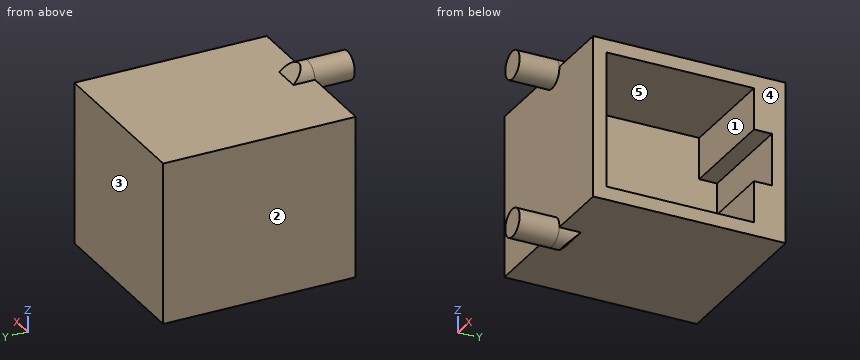
from build123d import *

# Parameters (mm, degrees)
SKETCH1_W           = 13
SKETCH1_H           = 12.2
BOSS_EXTRUDE1_DEPTH = 14.55
SKETCH2_R           = 1.05
BOSS_EXTRUDE2_DEPTH = 3
CUT_EXTRUDE1_DEPTH  = 8
CHAMFER1_SIZE       = 1.63


with BuildPart() as part:
    # Sketch1 → Boss-Extrude1 (new body)
    with BuildSketch(Plane(origin=(0, 0, 0), x_dir=(1, 0, 0), z_dir=(0, 1, 0))):
        with Locations((6.5, 6.1)):
            Rectangle(SKETCH1_W, SKETCH1_H)
    extrude(amount=BOSS_EXTRUDE1_DEPTH)

    # Sketch2 → Boss-Extrude2 (add)
    with BuildSketch(Plane.XZ):
        with Locations(Location((7, -0.1, 0), (0, 0, 174.5349762))):
            Circle(SKETCH2_R)
        with Locations(Location((7, -12.1, 0), (0, 0, 354.5349762))):
            Circle(SKETCH2_R)
    extrude(amount=BOSS_EXTRUDE2_DEPTH)

    # Sketch3 → Cut-Extrude1 (cut)
    with BuildSketch(Plane(origin=(13, 0, 0), x_dir=(0, 0, -1), z_dir=(1, 0, 0))):
        Polygon((1.000271868, 12.149637893), (1.000271868, 1.000271868), (11.199728132, 1.000271868), (11.199728132, 12.149637893), (8.065074736, 12.149637893), (8.065074736, 13.503489481), (4.134925264, 13.503489481), (4.134925264, 12.149637893), align=None)
    extrude(amount=-CUT_EXTRUDE1_DEPTH, mode=Mode.SUBTRACT)

    # Chamfer1
    # the kernel refuses this chamfer: 1.63 mm, written as the material it adds along each edge
    with BuildSketch(Plane(origin=(1.762929482, 0, 0), x_dir=(0, 0.9996219169112968, -0.027495876610586376), z_dir=(1, 0, 0))) as chamfer1_piece_1_section:
        Polygon((CHAMFER1_SIZE * 0.999621916911, CHAMFER1_SIZE * 0.0274958766106), (-CHAMFER1_SIZE * 0.0274958766106, CHAMFER1_SIZE * 0.999621916911), (0, 0), align=None)
    chamfer1_piece_1 = extrude(amount=10.474141037, mode=Mode.PRIVATE)
    chamfer1_piece_1 = chamfer1_piece_1 & Plane(origin=(7, 0.64054065, -0.1), x_dir=(-0.9954545219220755, 0, 0.09523809523973083), z_dir=(0, 1, 0)) * Cylinder(1.05, 28, mode=Mode.PRIVATE)
    add(chamfer1_piece_1)
    with BuildSketch(Plane(origin=(12.237070518, 0, -12.2), x_dir=(0, 0.9996219169112968, 0.02749587661058688), z_dir=(-1, 0, 0))) as chamfer1_piece_2_section:
        Polygon((CHAMFER1_SIZE * 0.999621916911, CHAMFER1_SIZE * 0.0274958766106), (-CHAMFER1_SIZE * 0.0274958766106, CHAMFER1_SIZE * 0.999621916911), (0, 0), align=None)
    chamfer1_piece_2 = extrude(amount=10.474141037, mode=Mode.PRIVATE)
    chamfer1_piece_2 = chamfer1_piece_2 & Plane(origin=(7, 0.64054065, -12.1), x_dir=(0.9954545219220756, 0, -0.09523809523973051), z_dir=(0, 1, 0)) * Cylinder(1.05, 28, mode=Mode.PRIVATE)
    add(chamfer1_piece_2)


solid = part.part
For this review, take the finished solid that the model builds, in its own axes (mm). Face numbers are marked on the shaded views. A direction names the side the tool comes from. Give positions to 0.01 mm unless a question says otherwise; leave off trailing zeros. Loops run counter-clockwise (first coordinate to the right, second up) from the corner with the lowest first, then second, coordinate; pieces in that order, holes last. Notation, with made-up numbers: (-22, 12) -> (0, 12) arc R11 ccw to (0, 30) -> close; hole circle Ø2 at (78.25, -21.75). An arc over 180 degrees is marked (long way). One line per question, with ' | ' between items.
1) We need section C-C (z = -8.75). Write out the cut boundary in (x, y), plus the area to 4 significant figures.
Resolved:
outline: (0, 0) -> (13, 0) -> (13, 1) -> (5, 1) -> (5, 12.15) -> (13, 12.15) -> (13, 14.55) -> (0, 14.55) -> close | area: 100.0 mm2
2) We need section A-A (x = 7). Write out the cut boundary in (y, z).
Resolved:
outline: (-3, -13.15) -> (0.68, -13.15) -> (1.63, -12.2) -> (14.55, -12.2) -> (14.55, 0) -> (1.63, 0) -> (0.68, 0.95) -> (-3, 0.95) -> (-3, -1.15) -> (0, -1.15) -> (0, -11.05) -> (-3, -11.05) -> close; hole (1, -11.2) -> (12.15, -11.2) -> (12.15, -8.07) -> (13.5, -8.07) -> (13.5, -4.13) -> (12.15, -4.13) -> (12.15, -1) -> (1, -1) -> close
3) For the marked faces 4 and 5, list the 3-axis set-ups (+Z, -Z, +X, -X, +Y, -Y) from which the entire face can be reached by the end or side of a thin tool; tool diameter is ignored.
Resolved:
face 4: +Z, -Z, +X, +Y, -Y | face 5: +X
4) We need section B-B (y = 4). Write out the cut boundary in (x, z), plus the area to 3 significant figures.
Resolved:
outline: (0, -12.2) -> (13, -12.2) -> (13, -11.2) -> (5, -11.2) -> (5, -1) -> (13, -1) -> (13, 0) -> (0, 0) -> close | area: 77.0 mm2
5) We need section D-D (y = -0.5). Write out the cut boundary in (x, z).
Resolved:
outline: circle Ø2.1 at (7, -12.1); circle Ø2.1 at (7, -0.1)
6) To check wall thickness, follow probe 1 along Y at (x, z) = (8.75, -11); probe 2 along Y at (x, z) = (8.5, -7.75); probe 3 along Z at (x, y) = (11, 9). State the ranges of each line that lie inside material, in increasing order.
Resolved:
probe 1: y = 0 to 1, 12.15 to 14.55 | probe 2: y = 0 to 1, 13.5 to 14.55 | probe 3: z = -12.2 to -11.2, -1 to 0
7) The part is to be moulded in two halves that separate along Y. For the marked faces 1, 2 and 3, say which applies: +Y half, -Y half, draft (parallel to the pull), parting line (faces both ways), or undercut.
Resolved:
face 1: undercut | face 2: draft | face 3: +Y half
8) Insertion check: pin 1 Ø0.9 at (x, z) = (8.5, -10) entering from -Y; pin 2 Ø5 at (x, y) = (1.5, -1) entering from -Z; pin 3 Ø2 at (y, z) = (5, -8.5) entering from +X. Each pin has a flat end and moves straight along its axis. Give the tip position at first contact, or say it passes through.
Resolved:
pin 1: stops at y = 0 | pin 2: stops at z = -12.2 | pin 3: stops at x = 5
